Verification items for the finished model (mm, model axes). A direction names the side the tool comes from. Give positions to 0.01 mm unless a question says otherwise; leave off trailing zeros. Loops run counter-clockwise (first coordinate to the right, second up) from the corner with the lowest first, then second, coordinate; pieces in that order, holes last. Notation, with made-up numbers: (27.25, 49.5) - (62.25, 49.5) arc R19 ccw to (62.25, 72.5) - close; hole circle Ø2 at (-33, -30). An arc over 180 degrees is marked (long way). Use one line per item in the form item = value.
```python
from build123d import *

# Parameters (mm, degrees)
SKETCH1_R           = 1.6
BOSS_EXTRUDE1_DEPTH = 3
CUT_EXTRUDE5_DEPTH  = 4
FILLET1_R           = 3.54


with BuildPart() as part:
    # Sketch1 → Boss-Extrude1 (new body)
    with BuildSketch(Plane.XY):
        with BuildLine():
            Line((-107, 98.923010333), (-107, -98.923010333))
            ThreePointArc((-107, -98.923010333), (-107.201661971, -101.11372249), (-107.799869959, -103.230804092))
            ThreePointArc((-107.799869959, -103.230804092), (-107, -107), (-103.230804092, -107.799869959))
            ThreePointArc((-103.230804092, -107.799869959), (-101.11372249, -107.201661971), (-98.923010333, -107))
            Line((-98.923010333, -107), (-43, -107))
            Line((-43, -107), (43, -107))
            Line((43, -107), (98.923010333, -107))
            ThreePointArc((98.923010333, -107), (101.11372249, -107.201661971), (103.230804092, -107.799869959))
            ThreePointArc((103.230804092, -107.799869959), (107, -107), (107.799869959, -103.230804092))
            ThreePointArc((107.799869959, -103.230804092), (107.201661971, -101.11372249), (107, -98.923010333))
            Line((107, -98.923010333), (107, 98.923010333))
            ThreePointArc((107, 98.923010333), (107.201661971, 101.11372249), (107.799869959, 103.230804092))
            ThreePointArc((107.799869959, 103.230804092), (107, 107), (103.230804092, 107.799869959))
            ThreePointArc((103.230804092, 107.799869959), (101.11372249, 107.201661971), (98.923010333, 107))
            Line((98.923010333, 107), (-98.923010333, 107))
            ThreePointArc((-98.923010333, 107), (-101.11372249, 107.201661971), (-103.230804092, 107.799869959))
            ThreePointArc((-103.230804092, 107.799869959), (-107, 107), (-107.799869959, 103.230804092))
            ThreePointArc((-107.799869959, 103.230804092), (-107.201661971, 101.11372249), (-107, 98.923010333))
        make_face()
        with Locations((-104.5, -104.5)):
            Circle(SKETCH1_R, mode=Mode.SUBTRACT)
        with Locations((-104.5, 104.5)):
            Circle(SKETCH1_R, mode=Mode.SUBTRACT)
        with Locations((104.5, 104.5)):
            Circle(SKETCH1_R, mode=Mode.SUBTRACT)
        with Locations((104.5, -104.5)):
            Circle(SKETCH1_R, mode=Mode.SUBTRACT)
    extrude(amount=BOSS_EXTRUDE1_DEPTH)

    # Sketch5 → Cut-Extrude5 (cut, through all)
    with BuildSketch(Plane.XY):
        with BuildLine():
            Line((-25.033358746, -107), (24.966641254, -107))
            Line((24.966641254, -107), (24.966641254, -69.5))
            ThreePointArc((24.966641254, -69.5), (23.50217516, -65.964466094), (19.966641254, -64.5))
            Line((19.966641254, -64.5), (12.966641254, -64.5))
            ThreePointArc((12.966641254, -64.5), (5.895573442, -61.571067812), (2.966641254, -54.5))
            Line((2.966641254, -54.5), (2.966641254, 0))
            ThreePointArc((2.966641254, 0), (-0.033358746, 3), (-3.033358746, 0))
            Line((-3.033358746, 0), (-3.033358746, -54.5))
            ThreePointArc((-3.033358746, -54.5), (-5.962290934, -61.571067812), (-13.033358746, -64.5))
            Line((-13.033358746, -64.5), (-20.033358746, -64.5))
            ThreePointArc((-20.033358746, -64.5), (-23.568892652, -65.964466094), (-25.033358746, -69.5))
            Line((-25.033358746, -69.5), (-25.033358746, -107))
        make_face()
    extrude(amount=CUT_EXTRUDE5_DEPTH, mode=Mode.SUBTRACT)

    # Fillet1
    fillet1_edges = [part.edges().sort_by_distance(p)[0] for p in [
        (-25.033358746, -107, 1.5),
        (24.966641254, -107, 1.5),
    ]]
    fillet(fillet1_edges, radius=FILLET1_R)


solid = part.part
```
1. Scan lines: probe 1 along X at (y, z) = (104.5, 1.9); probe 2 along X at (y, z) = (-17.5, 2.3). Record each from-to range of solid material in increasing order.
Result set:
probe_1 = -108.04 to -106.1, -102.9 to 102.9, 106.1 to 108.04
probe_2 = -107 to -3.03, 2.97 to 107
2. Section check B-B, the plane z = 1.1. State how many separate pieces and enclosed holes the cut face has, then the cut area to 3 significant figures.
Result set:
separate_pieces = 1
enclosed_holes = 4
area = 43,200 mm²
3. Section check A-A, the plane y = -87. Record the cut outline in (x, z).
Result set:
outline = (-107, 0) - (-25.03, 0) - (-25.03, 3) - (-107, 3) - close; (24.97, 0) - (107, 0) - (107, 3) - (24.97, 3) - close
4. Depth check by flat-ended pin: pin 1 Ø1.5 at (y, z) = (-93.5, 1.5) entering from +X; pin 2 Ø1 at (x, z) = (-20.5, 0.5) entering from +Y; pin 3 Ø0.9 at (x, z) = (15, 1) entering from -Y. Enter the tip coordinate at first touch or a pass-through.
Result set:
pin_1 = 107
pin_2 = 107
pin_3 = -64.5
5. Tool access check on faces 3 (the flat face through (-2, 26, 3)), 4 (the cylindrical face through (5.974, -61.648, 1.479)). Record the directions out of +Z, -Z, +X, -X, +Y, -Y that give a thin tool (end or side, any length) a straight path to the whole face; none if there is none.
Result set:
face_3 = +Z, +X, -X, +Y, -Y
face_4 = +Z, -Z, -Y
6. Draft check along X on faces 1 (the flat face through (-2, 26, 0)), 2 (the cylindrical face through (-23.53, -65.926, 1.479)). Enter one of: released by +X, released by -X, zero draft, split by the parting line, or undercut.
Result set:
face_1 = zero draft
face_2 = undercut
7. Section check C-C, the plane y = -43. Record the cut outline in (x, z).
Result set:
outline = (-107, 0) - (-3.03, 0) - (-3.03, 3) - (-107, 3) - close; (2.97, 0) - (107, 0) - (107, 3) - (2.97, 3) - close
